```python
from build123d import *

# Parameters (mm, degrees)
SKIZZE1_R                       = 5
SKIZZE1_R_2                     = 4
AUFSATZ_LINEAR_AUSTRAGEN1_DEPTH = 100
BOSS_EXTRUDE2_REACH             = 103.242
BOSS_EXTRUDE2_END_RADIUS        = 5
SKETCH1_W                       = 5
SKETCH1_H                       = 5


with BuildPart() as part:
    # Skizze1 → Aufsatz-Linear austragen1 (new body)
    with BuildSketch(Plane.XY):
        Circle(SKIZZE1_R)
        Circle(SKIZZE1_R_2, mode=Mode.SUBTRACT)
    extrude(amount=AUFSATZ_LINEAR_AUSTRAGEN1_DEPTH)

    # Boss-Extrude2: up to this cylinder (the profile starts outside it)
    boss_extrude2_end = Plane(origin=(0, 0, 50), z_dir=(0, 0, -1)) * Cylinder(BOSS_EXTRUDE2_END_RADIUS, 217.484, mode=Mode.PRIVATE)
    # Sketch1 → Boss-Extrude2 (add, up to the surface)
    with BuildSketch(Plane(origin=(10, 0, 0), x_dir=(0, 0, -1), z_dir=(1, 0, 0)), mode=Mode.PRIVATE) as boss_extrude2_sk1:
        with Locations((-50, 0)):
            Rectangle(SKETCH1_W, SKETCH1_H)
    boss_extrude2_tool1 = extrude(boss_extrude2_sk1.sketch, amount=-BOSS_EXTRUDE2_REACH, mode=Mode.PRIVATE) - boss_extrude2_end
    add(boss_extrude2_tool1.solids().sort_by_distance((10, 0, 50))[0])


solid = part.part
```
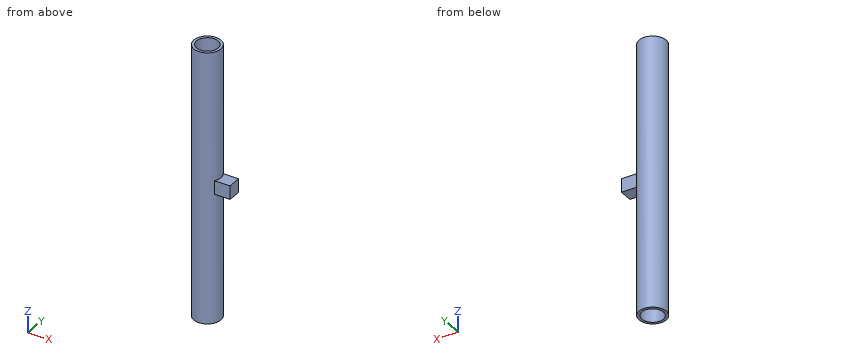
Input: part model. Units: mm. Frame: model coordinates. Coordinates: 2 decimals unless noted, no trailing zeros. Loops run counter-clockwise (first coordinate to the right, second up) from the corner with the lowest first, then second, coordinate; pieces in that order, holes last.
Q1. Line query: line 1 along Y through (x, z) = (0, 70); line 2 along X through (y, z) = (2.25, 45); line 3 along X through (y, z) = (1.5, 66). Output: solid intervals per line, ascending.
Results are:
line 1: y = -5 to -4, 4 to 5
line 2: x = -4.47 to -3.31, 3.31 to 4.47
line 3: x = -4.77 to -3.71, 3.71 to 4.77
Q2. Section A-A, the plane x = 0. Return the cut outline in (y, z), and give its area (3 significant figures).
Results are:
outline: (-5, 0) - (-4, 0) - (-4, 100) - (-5, 100) - close; (4, 0) - (5, 0) - (5, 100) - (4, 100) - close
area: 200 mm2
Q3. Contact query for flat-ended pins moving along their axis: pin 1 (1.5 mm diameter, centred on x = 6.5, z = 75, fed in from -Y); pin 2 (2.5 mm diameter, centred on x = 7, z = 50.5, fed in from +Y); pin 3 (4 mm diameter, centred on y = -3.5, z = 65.5, fed in from -X); pin 4 (4 mm diameter, centred on x = 8, y = -1, fed in from -Z). Output: stop coordinate, or through.
Results are:
pin 1: passes through
pin 2: stops at y = 2.5
pin 3: stops at x = -4.77
pin 4: stops at z = 47.5
Q4. Section C-C, the plane z = 7.5. Return the cut outline in (x, y).
Results are:
outline: circle Ø10 at (0, 0); hole circle Ø8 at (0, 0)
Q5. Section B-B, the plane y = 0. Return the cut outline in (x, z), and give its area (3 significant figures).
Results are:
outline: (-5, 0) - (-4, 0) - (-4, 100) - (-5, 100) - close; (4, 0) - (5, 0) - (5, 47.5) - (10, 47.5) - (10, 52.5) - (5, 52.5) - (5, 100) - (4, 100) - close
area: 225 mm2
Q6. Section D-D, the plane x = 6.25. Return the cut outline in (y, z).
Results are:
outline: (-2.5, 47.5) - (2.5, 47.5) - (2.5, 52.5) - (-2.5, 52.5) - close
